Source: CAD feature listing. Evaluate the final solid. Frame: model axes, mm. A direction names the side the tool comes from. Give positions to 0.01 mm unless a question says otherwise; leave off trailing zeros. Order: outer loops, then holes, each group sorted by start corner. A loop starts at its lowest first (then second) coordinate and runs counter-clockwise, first axis right, second up.
1) First-contact query: P1, Ø1.5, axis at x = 6, z = -9.5, coming from the -Y side; P2, Ø1, axis at x = 2, z = 9.5, coming from the -Y side; P3, Ø2, axis at y = -12.5, z = 9, coming from the +X side. Flat tips, straight axial feed; report the tip coordinate or a pass-through.
2) Material intervals for line 1 (X direction, y = -15.5, z = 6.25); line 2 (X direction, y = 5.75, z = -8.85); line 3 (X direction, y = 2.5, z = -8.85), sorted ascending.
3) Draft query along X for faces 5 (the face through (-34, -7, 0)), 6 (the face through (0, 6, 12)), 7 (the face through (20.46, 5.58, 9.31)). Return one class per face: released by +X, released by -X, zero draft, split by the parting line, or undercut.
4) Section A-A, the plane y = -13.5. Return loops of the section in (x, z), plus the area to 3 significant figures.
5) Section B-B, the plane z = 0. Return loops of the section in (x, y).
6) Access query for faces 1 (the face through (-6, 2, -9)), 2 (the face through (29, -6, -9.5)), 3 (the face through (-29, -6, 9.5)), 4 (the face through (19.8, 11.51, -8.04)). Directions: +Z, -Z, +X, -X, +Y, -Y. A direction counts if a zero-diameter tool reaches every point of the face in a straight line with its end or side. Return the directions, or none.
7) Section D-D, the plane y = 1.5. Give the number of separate pieces and of enclosed holes in the cut face, plus the area to 4 significant figures.
8) Section C-C, the plane x = -12.75. Return loops of the section in (y, z).
```python
from build123d import *

# Parameters (mm, degrees)
SKETCH1_W                = 52
SKETCH1_H                = 24
SKETCH1_R                = 8.25
BOSS_EXTRUDE1_DEPTH      = 12
SKETCH2_R                = 1
CUT_EXTRUDE1_DEPTH       = 32.048349393
SKETCH3_R                = 1.75
CUT_EXTRUDE2_DEPTH       = 1
CUT_EXTRUDE3_DEPTH       = 5
FILLET3_R                = 0.5
CHAMFER1_SIZE            = 2.5
SKETCH5_W                = 19
SKETCH5_H                = 12
BOSS_EXTRUDE2_DEPTH      = 8
SKETCH6_W                = 7
SKETCH6_H                = 19
BOSS_EXTRUDE3_DEPTH      = 24
CHAMFER2_SIZE            = 3
CHAMFER2_OF_MIRROR1_SIZE = 3
SKETCH7_W                = 14
SKETCH7_H                = 8
CUT_EXTRUDE4_DEPTH       = 5
FILLET4_R                = 0.5


with BuildPart() as part:
    # Sketch1 → Boss-Extrude1 (new body)
    with BuildSketch(Plane(origin=(0, 0, 0), x_dir=(1, 0, 0), z_dir=(0, 1, 0))):
        Rectangle(SKETCH1_W, SKETCH1_H)
        with Locations(Location((12.75, 0, 0), (0, 0, 270))):
            Circle(SKETCH1_R, mode=Mode.SUBTRACT)
        with Locations(Location((-12.75, 0, 0), (0, 0, 270))):
            Circle(SKETCH1_R, mode=Mode.SUBTRACT)
    extrude(amount=BOSS_EXTRUDE1_DEPTH)

    # Sketch2 → Cut-Extrude1 (cut, through all)
    with BuildSketch(Plane(origin=(0, 12, 0), x_dir=(1, 0, 0), z_dir=(0, 1, 0))):
        with Locations(Location((-21.35, 8.85, 0), (0, 0, 270))):
            Circle(SKETCH2_R)
        with Locations(Location((21.35, 8.85, 0), (0, 0, 270))):
            Circle(SKETCH2_R)
        with Locations(Location((21.35, -8.85, 0), (0, 0, 270))):
            Circle(SKETCH2_R)
        with Locations(Location((-21.35, -8.85, 0), (0, 0, 270))):
            Circle(SKETCH2_R)
    extrude(amount=-CUT_EXTRUDE1_DEPTH, mode=Mode.SUBTRACT)

    # Sketch3 → Cut-Extrude2 (cut)
    with BuildSketch(Plane(origin=(0, 12, 0), x_dir=(1, 0, 0), z_dir=(0, 1, 0))):
        with Locations(Location((-21.35, 8.85, 0), (0, 0, 270))):
            Circle(SKETCH3_R)
        with Locations(Location((21.35, 8.85, 0), (0, 0, 270))):
            Circle(SKETCH3_R)
        with Locations(Location((21.35, -8.85, 0), (0, 0, 270))):
            Circle(SKETCH3_R)
        with Locations(Location((-21.35, -8.85, 0), (0, 0, 270))):
            Circle(SKETCH3_R)
    extrude(amount=-CUT_EXTRUDE2_DEPTH, mode=Mode.SUBTRACT)

    # Sketch4 → Cut-Extrude3 (cut)
    with BuildSketch(Plane.XZ):
        Polygon((-6, -5), (-6, -12), (6, -12), (6, -5), (0, -5), align=None)
    extrude(amount=-CUT_EXTRUDE3_DEPTH, mode=Mode.SUBTRACT)

    # Fillet3
    fillet3_edges = [part.edges().sort_by_distance(p)[0] for p in [
        (-6, 2.5, -5),
        (6, 5, -8.5),
        (6, 2.5, -5),
        (-6, 5, -8.5),
        (0, 5, -5),
    ]]
    fillet(fillet3_edges, radius=FILLET3_R)

    # Chamfer1
    chamfer1_edges = [part.edges().sort_by_distance(p)[0] for p in [
        (26, 6, 12),
        (-26, 6, 12),
        (-26, 6, -12),
        (26, 6, -12),
    ]]
    chamfer(chamfer1_edges, length=CHAMFER1_SIZE)

    # Sketch5 → Boss-Extrude2 (add)
    with BuildSketch(Plane.ZY.offset(26)):
        with Locations((0, 6)):
            Rectangle(SKETCH5_W, SKETCH5_H)
    boss_extrude2 = extrude(amount=BOSS_EXTRUDE2_DEPTH)

    # Sketch6 → Boss-Extrude3 (add)
    with BuildSketch(Plane.XZ):
        with Locations((-30.5, 0)):
            Rectangle(SKETCH6_W, SKETCH6_H)
    boss_extrude3 = extrude(amount=BOSS_EXTRUDE3_DEPTH)

    # Chamfer2
    chamfer2_edges = [part.edges().sort_by_distance(p)[0] for p in [
        (-34, -6, 9.5),
        (-34, 12, 0),
        (-34, -6, -9.5),
    ]]
    chamfer(chamfer2_edges, length=CHAMFER2_SIZE)

    # Mirror1: Boss-Extrude2, Boss-Extrude3 across plane
    add(boss_extrude2.mirror(Plane(origin=(0, 0, 0), x_dir=(0, 0, 1), z_dir=(1, 0, 0))))
    add(boss_extrude3.mirror(Plane(origin=(0, 0, 0), x_dir=(0, 0, 1), z_dir=(1, 0, 0))))

    # Chamfer2 of Mirror1
    chamfer2_of_mirror1_edges = [part.edges().sort_by_distance(p)[0] for p in [
        (34, -6, 9.5),
        (34, 12, 0),
        (34, -6, -9.5),
    ]]
    chamfer(chamfer2_of_mirror1_edges, length=CHAMFER2_OF_MIRROR1_SIZE)

    # Sketch7 → Cut-Extrude4 (cut)
    with BuildSketch(Plane.XZ):
        with Locations((0, 12)):
            Rectangle(SKETCH7_W, SKETCH7_H)
    extrude(amount=-CUT_EXTRUDE4_DEPTH, mode=Mode.SUBTRACT)

    # Fillet4
    fillet4_edges = [part.edges().sort_by_distance(p)[0] for p in [
        (-7, 2.5, 8),
        (7, 5, 10),
        (0, 5, 8),
        (-7, 5, 10),
        (7, 2.5, 8),
    ]]
    fillet(fillet4_edges, radius=FILLET4_R)


solid = part.part
```
From the geometry:
1. P1: stops at y = 0
1. P2: stops at y = 5
1. P3: stops at x = 32.5
2. line 1: x = -34 to -27, 27 to 34
2. line 2: x = -31.65 to -22.35, -20.35 to 20.35, 22.35 to 31.65
2. line 3: x = -31.65 to -22.35, -20.35 to -6, 6 to 20.35, 22.35 to 31.65
3. face 5: released by -X
3. face 6: zero draft
3. face 7: undercut
4. outline: (-34, -6.5) - (-31, -9.5) - (-27, -9.5) - (-27, 9.5) - (-31, 9.5) - (-34, 6.5) - close; (27, -9.5) - (31, -9.5) - (34, -6.5) - (34, 6.5) - (31, 9.5) - (27, 9.5) - close
4. area: 248 mm2
5. outline: (-34, -24) - (-27, -24) - (-27, 0) - (-21, 0) - (-21, 12) - (-31, 12) - (-34, 9) - close; (-4.5, 0) - (4.5, 0) - (4.5, 12) - (-4.5, 12) - close; (21, 0) - (27, 0) - (27, -24) - (34, -24) - (34, 9) - (31, 12) - (21, 12) - close
6. face 1: -Z, -Y
6. face 2: -Z, +X, +Y, -Y
6. face 3: +Z, -X, +Y, -Y
6. face 4: +Y
7. separate pieces: 1
7. enclosed holes: 6
7. area: 941.5 mm2
8. outline: (0, -12) - (12, -12) - (12, -8.25) - (0, -8.25) - close; (0, 8.25) - (12, 8.25) - (12, 12) - (0, 12) - close
